```python
from build123d import *

# Parameters (mm, degrees)
BOSS_EXTRUDE1_DEPTH = 31.75
CUT_EXTRUDE1_REACH  = 6.762
SKETCH5_R           = 3.2639


with BuildPart() as part:
    # Sketch2 → Boss-Extrude1 (new body, symmetric)
    with BuildSketch(Plane.XY):
        with BuildLine():
            Line((-19.05, -19.05), (19.05, -19.05))
            Line((19.05, -19.05), (19.05, 19.05))
            Line((19.05, 19.05), (16.66875, 19.05))
            ThreePointArc((16.66875, 19.05), (14.984951977, 18.352548023), (14.2875, 16.66875))
            Line((14.2875, 16.66875), (14.2875, -9.5123))
            ThreePointArc((14.2875, -9.5123), (12.888876302, -12.888876302), (9.5123, -14.2875))
            Line((9.5123, -14.2875), (-16.66875, -14.2875))
            ThreePointArc((-16.66875, -14.2875), (-18.352548023, -14.984951977), (-19.05, -16.66875))
            Line((-19.05, -16.66875), (-19.05, -19.05))
        make_face()
    extrude(amount=BOSS_EXTRUDE1_DEPTH, both=True)

    # Sketch5 → Cut-Extrude1 (cut, up to next)
    with BuildSketch(Plane.ZY.offset(-14.2875), mode=Mode.PRIVATE) as cut_extrude1_sk1:
        with Locations((-19.05, 6.35)):
            Circle(SKETCH5_R)
    cut_extrude1_tool1 = extrude(cut_extrude1_sk1.sketch, amount=-CUT_EXTRUDE1_REACH, mode=Mode.PRIVATE) & part.part
    add(cut_extrude1_tool1.solids().sort_by_distance((14.2875, 6.35, -19.05))[0], mode=Mode.SUBTRACT)
    # Sketch5 → Cut-Extrude1 (cut, up to next)
    with BuildSketch(Plane.ZY.offset(-14.2875), mode=Mode.PRIVATE) as cut_extrude1_sk2:
        with Locations((19.05, 6.35)):
            Circle(SKETCH5_R)
    cut_extrude1_tool2 = extrude(cut_extrude1_sk2.sketch, amount=-CUT_EXTRUDE1_REACH, mode=Mode.PRIVATE) & part.part
    add(cut_extrude1_tool2.solids().sort_by_distance((14.2875, 6.35, 19.05))[0], mode=Mode.SUBTRACT)


solid = part.part
```
CAD build for the part. Positions are in the model's coordinates, mm. A direction names the side the tool comes from. Give positions to 0.01 mm unless a question says otherwise; leave off trailing zeros. Order: outer loops, then holes, each group sorted by start corner. A loop starts at its lowest first (then second) coordinate and runs counter-clockwise, first axis right, second up. Notation, with made-up numbers: M 21,26.5 L 65,26.5 A9 ccw 65,37.5 Z; hole C 47.5,52.5 d8. An arc over 180 degrees is marked long. Put each result on its own line as item: value. Start each with the question number.
(1) Saw through at C-C, the plane z = -5.5. Write the cut outline in (x, y), then the cut area to 3 significant figures.
(2) Mould opens along Z. For faces 3 (the cylindrical face through (16.635, 5.1, 22.065)), 4 (the flat face through (19.05, 0, 0)), 5 (the flat face through (8, -15, 31.75)) say: +Z half, -Z half, draft (parallel to the pull), parting line (faces both ways), or undercut.
(3) Saw through at A-A, the plane z = -19.05. Write the cut outline in (x, y).
(4) Drill centre lines: line 1 along Y through (x, z) = (17.75, -19.05); line 2 along Z through (x, y) = (17, 6); line 3 along X through (y, z) = (6, -11). Where is each one in solid material? Low to high.
(5) Flat gauge pins, fed straight in: pin 1 Ø5 at (y, z) = (-5, -10) entering from -X; pin 2 Ø2 at (x, z) = (11.5, 3) entering from +Y. Where does each tip first touch, or does it go through?
(6) Saw through at B-B, the plane y = 6.35. Write the cut outline in (x, z).
(7) Which spindle directions (+Z, -Z, +X, -X, +Y, -Y) get a long thin tool onto all of the face, cutting with end or side? Do faces 1 (the cylindrical face through (16.64, 6.49, -22.31)), 2 (the flat face through (-3, -14.288, 0)). Say none if no direction does.
(8) Saw through at D-D, the plane x = -10. Write the cut outline in (y, z), then the cut area to 3 significant figures.
Check result:
1. outline: M -19.05,-19.05 L 19.05,-19.05 L 19.05,19.05 L 16.67,19.05 A2.38 ccw 14.29,16.67 L 14.29,-9.51 A4.78 cw 9.51,-14.29 L -16.67,-14.29 A2.38 ccw -19.05,-16.67 Z
1. area: 343 mm2
2. face 3: undercut
2. face 4: draft
2. face 5: +Z half
3. outline: M -19.05,-19.05 L 19.05,-19.05 L 19.05,3.09 L 14.29,3.09 L 14.29,-9.51 A4.78 cw 9.51,-14.29 L -16.67,-14.29 A2.38 ccw -19.05,-16.67 Z; M 14.29,9.61 L 19.05,9.61 L 19.05,19.05 L 16.67,19.05 A2.38 ccw 14.29,16.67 Z
4. line 1: y = -19.05 to 3.09, 9.61 to 19.05
4. line 2: z = -31.75 to -22.3, -15.8 to 15.8, 22.3 to 31.75
4. line 3: x = 14.29 to 19.05
5. pin 1: stops at x = 14.29
5. pin 2: stops at y = -13.24
6. outline: M 14.29,-31.75 L 19.05,-31.75 L 19.05,-22.31 L 14.29,-22.31 Z; M 14.29,-15.79 L 19.05,-15.79 L 19.05,15.79 L 14.29,15.79 Z; M 14.29,22.31 L 19.05,22.31 L 19.05,31.75 L 14.29,31.75 Z
7. face 1: +X, -X
7. face 2: +Z, -Z, -X, +Y
8. outline: M -19.05,-31.75 L -14.29,-31.75 L -14.29,31.75 L -19.05,31.75 Z
8. area: 302 mm2
